```python
from build123d import *

# Parameters (mm, degrees)
F0_W     = 100
F0_H     = 50
F1_DEPTH = 25


with BuildPart() as f1:
    # F0 (on Top) → F1 (new body)
    with BuildSketch(Plane.XY):
        Rectangle(F0_W, F0_H)
    extrude(amount=F1_DEPTH)

    # F2 (on face) → F3 (revolve, cut)
    with BuildSketch(Plane.XY.offset(25)):
        with BuildLine():
            Line((-17.400011, 16), (-32.400011, 16))
            ThreePointArc((-32.400011, 16), (-35.935545, 14.535534), (-37.400011, 11))
            Line((-37.400011, 11), (-37.400011, 0))
            Line((-37.400011, 0), (36.599989, 0))
            Line((36.599989, 0), (36.599989, 6.097698))
            ThreePointArc((36.599989, 6.097698), (34.831864, 9.912798), (30.777994, 11.029668))
            Line((30.777994, 11.029668), (6.599989, 7))
            Line((6.599989, 7), (-9.400011, 7))
            Line((-9.400011, 7), (-17.400011, 16))
        make_face()
    revolve(axis=Axis((1.115499, 0, 25), (1, 0, 0)), mode=Mode.SUBTRACT)


solid = f1.part
```
The model under review builds one solid part; all positions refer to its coordinate system, in mm. A direction names the side the tool comes from. Round coordinates to 2 decimals unless told otherwise and drop trailing zeros. Write each loop counter-clockwise with the first axis right and the second up, starting at its lowest first coordinate (ties: lowest second). Pieces come first, ordered by that corner, then holes. Notation, with made-up numbers: M 49,15.5 L 92,15.5 A22 cw 92,29.5 Z; hole C 84,59.5 d11. An arc over 180 degrees is marked long. Use CSV: the item, a comma, the result in double quotes. Start each with the question number.
(1) We need section A-A, the plane x = 18. State the section outline as (y, z) points, then the cut area to 3 significant figures.
(2) We need section B-B, the plane y = 0. State the section outline as (x, z) points, then the cut area to 3 significant figures.
(3) The part is to be moulded in two halves that separate along X. For faces 3 (the face through (-1, 0, 0)), 4 (the face through (-50, 0, 12)), 5 (the face through (18.52, -0.198, 16.016)), say which applies: +X half, -X half, draft (parallel to the pull), parting line (faces both ways), or undercut.
(4) Tool access review of faces 1 (the face through (-1, 11, 25)), 2 (the face through (36.6, 0, 23)): name each direction out of +Z, -Z, +X, -X, +Y, -Y from which nothing blocks a thin tool from reaching the whole face with its end or side.
(5) For line 1 along Z through (x, y) = (-29, 0.5); line 2 along X through (y, z) = (9, 17.25); line 3 along Y through (x, z) = (-11.5, 24), list the stretches that pass through material, from the lowest coordinate up.
(6) We need section C-C, the plane z = 16. State how many separate pieces and enclosed holes the cut face has, then the cut area to 3 significant figures.
Findings:
1,outline,"M -25,0 L 25,0 L 25,25 L 8.9,25 A8.9 cw -8.9,25 L -25,25 Z"
1,area,"1,130 mm^2"
2,outline,"M -50,0 L 50,0 L 50,25 L 36.6,25 L 36.6,18.9 A5 cw 30.78,13.97 L 6.6,18 L -9.4,18 L -17.4,9 L -32.4,9 A5 cw -37.4,14 L -37.4,25 L -50,25 Z"
2,area,"1,700 mm^2"
3,face 3,"draft"
3,face 4,"-X half"
3,face 5,"undercut"
4,face 1,"+Z, +X, -X, +Y, -Y"
4,face 2,"+Z"
5,line 1,"0 to 9.01"
5,line 2,"-50 to -37.32, -13.74 to 50"
5,line 3,"-25 to -9.31, 9.31 to 25"
6,separate pieces,"1"
6,enclosed holes,"2"
6,area,"4,230 mm^2"
